Can you work these out from the drawing? Everything is in mm from the part's minimum corner. A direction names the side the tool comes from. Coordinates: 2 decimals unless noted, no trailing zeros. Loops run counter-clockwise (first coordinate to the right, second up) from the corner with the lowest first, then second, coordinate; pieces in that order, holes last.
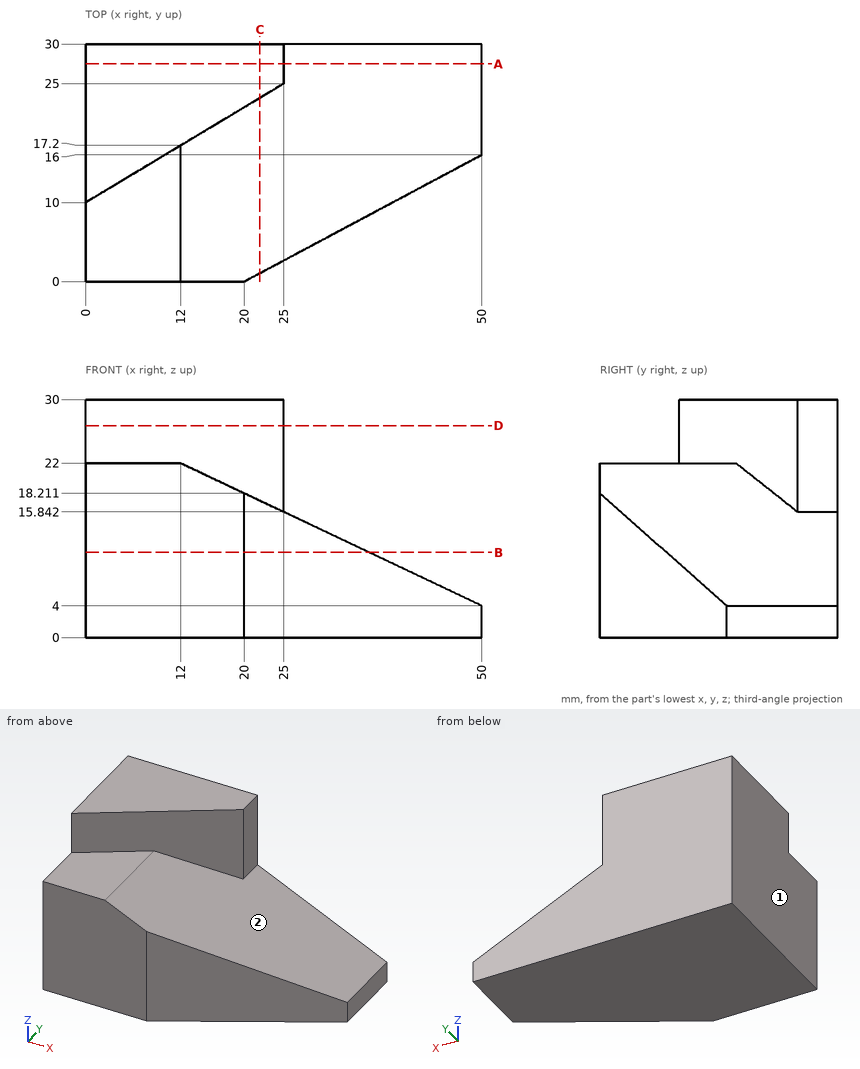
(1) Imagine slicing it at B-B, the plane z = 10.75. Write out the boundary of the cut face in (x, y), and give its area (3 significant figures).
Answers:
outline: (0, 0) - (20, 0) - (35.75, 8.4) - (35.75, 30) - (0, 30) - close
area: 1,010 mm2
(2) Imagine slicing it at A-A, the plane y = 27.5. Write out the boundary of the cut face in (x, z), and give its area (3 significant figures).
Answers:
outline: (0, 0) - (50, 0) - (50, 4) - (25, 15.84) - (25, 30) - (0, 30) - close
area: 998 mm2
(3) I need wall thicknesses on probe 1 along Z at (x, y) = (6, 12.5); probe 2 along X at (y, z) = (16, 25.5); probe 3 along Y at (x, z) = (20, 26.75). Which ranges of each line are inside material? Lowest first, please.
Answers:
probe 1: z = 0 to 22
probe 2: x = 0 to 10
probe 3: y = 22 to 30
(4) Imagine slicing it at D-D, the plane z = 26.75. Write out the boundary of the cut face in (x, y).
Answers:
outline: (0, 10) - (25, 25) - (25, 30) - (0, 30) - close
(5) Which directions (+Z, -Z, +X, -X, +Y, -Y) give clear straight access to the entire face, cutting with the end or side of a thin tool? Please do the marked faces 1 and 2.
Answers:
face 1: +Z, -Z, -X, +Y, -Y
face 2: +Z, +X, -Y
(6) For pin 1 (5.5 mm diameter, centred on y = 28, z = 24, fed in from +X); pin 2 (5 mm diameter, centred on x = 38, y = 23, fed in from +Z); pin 3 (5 mm diameter, centred on x = 28, z = 23, fed in from +Y); pin 4 (1 mm diameter, centred on y = 13.5, z = 20, fed in from +X) (1 decimal), each with a flat end and sliding along its axis, tell me the tip position at first contact or that it passes through.
Answers:
pin 1: stops at x = 25
pin 2: stops at z = 10.87
pin 3: passes through
pin 4: stops at x = 17.3
(7) Imagine slicing it at C-C, the plane x = 22. Write out the boundary of the cut face in (y, z), and give its area (3 significant figures).
Answers:
outline: (1.07, 0) - (30, 0) - (30, 30) - (23.2, 30) - (23.2, 17.26) - (1.07, 17.26) - close
area: 586 mm2
